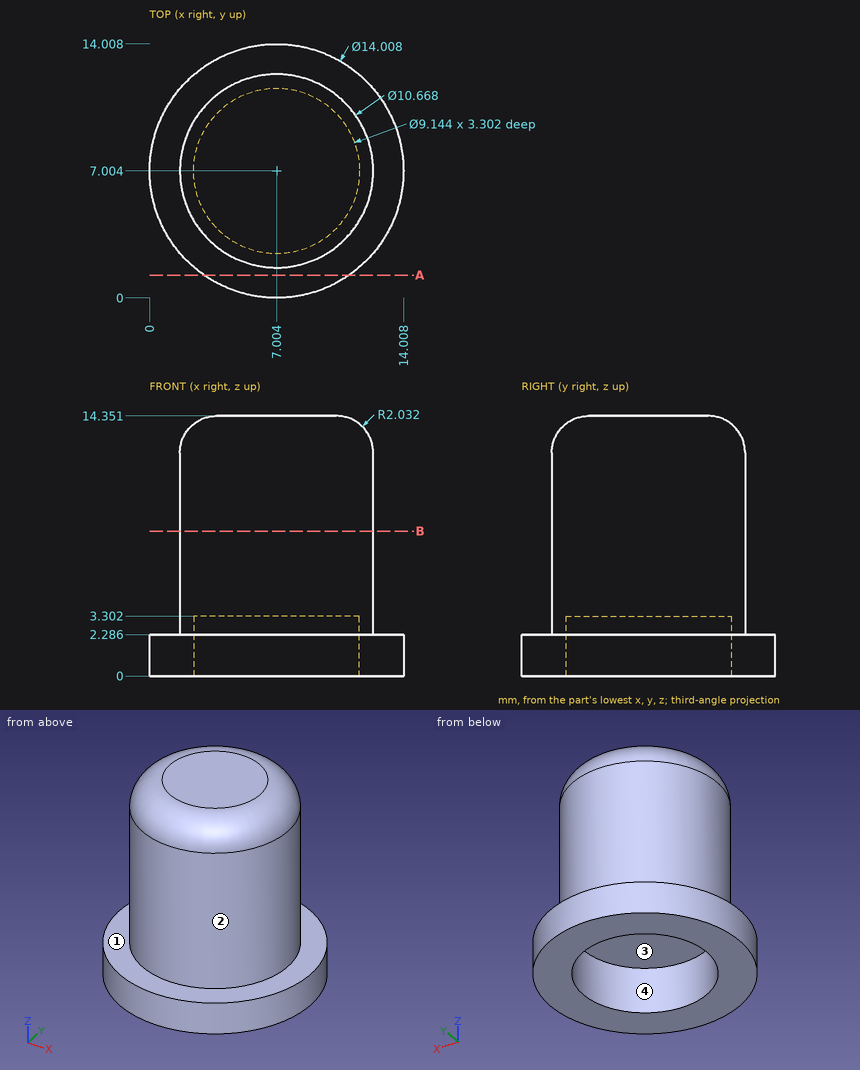
Here's the drawing with two shaded views (mm, measured from the low corner). I have some questions. Give positions to 0.01 mm unless a question says otherwise; leave off trailing zeros. Write each loop counter-clockwise with the first axis right and the second up, starting at its lowest first coordinate (ties: lowest second). Pieces come first, ordered by that corner, then holes. Notation, with made-up numbers: (47.5, -18.75) -> (57.5, -18.75) arc R26 cw to (57.5, -3.75) -> close; hole circle Ø11 at (-27, 4). An arc over 180 degrees is marked (long way). Answer as a JSON object with one key per item and string values. Group by question number.
Item 1: Suppose I cut it at A-A (y = 1.25). Please give me the cut outline in (x, z).
Item 2: We'd pull the mould along X, two halves only. Please class the marked faces 1, 2, 3 and 4: +X half, -X half, draft (parallel to the pull), parting line (faces both ways), or undercut.
Item 3: Suppose I cut it at B-B (z = 8). Please give me the cut outline in (x, y), plus the area to 3 significant figures.
Item 4: I'm going to push flat-ended pins straight in: P1, Ø4, axis at x = 9, z = 9, coming from the +Y side; P2, Ø1, axis at x = 3.5, z = 9.5, coming from the +Y side; P3, Ø8, axis at x = 11.5, z = 5, coming from the -Y side (1 decimal). Where does each tip first touch, or does it pass through?
Item 5: Please list where these lines run through material, in increasing order: line 1 (Z direction, x = 12, y = 9.75); line 2 (Z direction, x = 5.75, y = 8.5); line 3 (X direction, y = 9.75, z = 11) (1 decimal). Write a range as [from, to].
Findings:
{
 "1": {"outline": "(3.01, 0) -> (11, 0) -> (11, 2.29) -> (3.01, 2.29) -> close"},
 "2": {"face 1": "draft", "face 2": "parting line", "face 3": "undercut", "face 4": "undercut"},
 "3": {"outline": "circle Ø10.67 at (7, 7)", "area": "89.4 mm²"},
 "4": {"P1": "stops at y = 12.34", "P2": "stops at y = 11.41", "P3": "stops at y = 0.2"},
 "5": {"line 1": "z = [0, 2.29]", "line 2": "z = [3.3, 14.35]", "line 3": "x = [2.4, 11.6]"}
}
